Autodesk Fusion 360 part; units mm, degrees
sketch "Skizze1" plane through (0, 0, 0) normal (0, 0, 1) x (1, 0, 0)
  line L0 (-31.5508, 0) -> (33.8224, 0) construction
  line L1 (0, 25.6192) -> (0, -38.4919) construction
  circle A0 centre (0, 0) radius 1.75
  circle A1 centre (0, 0) radius 3.5
  circle A2 centre (0, 0) radius 5
  dimension "d1" = 3.5
  dimension "d2" = 7
  dimension "d3" = 10
extrude "Extrusion1" add sketch "Skizze1" along normal blind 7 contours A1 | A2
extrude "Extrusion2" add sketch "Skizze1" along normal blind 9.5 contours A1
ref_plane "Arbeitsebene1" through (0, 0, 3.5) normal (0, 0, 1) x (1, 0, 0)
sketch "Skizze2" plane through (0, 0, 3.5) normal (0, 0, 1) x (1, 0, 0)
  line L0 (-11, 0) -> (19, 0) construction
  line L1 (0, 16) -> (0, -23) construction
  line L2 (1.6743, -2.9) -> (3.3486, 0)
  line L3 (3.3486, 0) -> (1.6743, 2.9)
  line L4 (1.6743, 2.9) -> (-1.6743, 2.9)
  line L5 (-1.6743, 2.9) -> (-3.3486, 0)
  line L6 (-3.3486, 0) -> (-1.6743, -2.9)
  line L7 (-1.6743, -2.9) -> (1.6743, -2.9)
  dimension "d9" = 5.8
extrude "Extrusion3" cut sketch "Skizze2" along normal mid plane 2.8
Can you work these out from the model? Positions are in its coordinate system, mm. A direction names the side the tool comes from. Round coordinates to 2 decimals unless told otherwise and drop trailing zeros. Write each loop counter-clockwise with the first axis right and the second up, starting at its lowest first coordinate (ties: lowest second). Pieces come first, ordered by that corner, then holes. Notation, with made-up numbers: (85.5, 75) -> (129.5, 75) arc R24 ccw to (129.5, 96) -> close; hole circle Ø9 at (4, -9.75). An arc over 180 degrees is marked (long way). One line per question, with ' | ' between items. Start each with the question number.
1) I need wall thicknesses on line 1 (Y direction, x = 0, z = 0.65); line 2 (X direction, y = 0, z = 7.1). Which ranges of each line are inside material? Lowest first, please. Write a range as [from, to].
2) Suppose I cut it at D-D on x = -4. Write out the boundary of the cut face in (y, z), then the cut area to 3 significant figures.
3) If we mould it in two halves opening along Y, with no side actions, what happens to faces 4 (the flat face through (2, 0, 0)), 5 (the cylindrical face through (-1.08, 4.88, 3.45)), 6 (the flat face through (0, -2.9, 3))? For each: released by +Y, released by -Y, zero draft, split by the parting line, or undercut.
4) On a 3-axis mill with a long thin cutter (end or side, diameter ignored), from which of +Z, -Z, +X, -X, +Y, -Y can I reach the whole of each face in a straight line? I mean faces 1 (the flat face through (2.5, -1.47, 3.48)), 2 (the cylindrical face through (1.617, 0.67, 1.035)), 3 (the flat face through (2.2, -3.3, 7)). Say none if no direction works.
5) Suppose I cut it at C-C on y = -0.75. Write out the boundary of the cut face in (x, z), then the cut area to 3 significant figures.
6) Suppose I cut it at A-A on x = 0. Write out the boundary of the cut face in (y, z).
7) I'm going to push flat-ended pins straight in: P1, Ø1, axis at x = 3, y = 3, coming from the +Z side; P2, Ø3, axis at x = -2, z = 6, coming from the -Y side; P3, Ø2, axis at x = 3.5, z = 3.5, coming from the +Y side. Where does each tip first touch, or does it pass through?
8) Suppose I cut it at B-B on z = 4.75. Write out the boundary of the cut face in (x, y).
Return value:
1) line 1: y = [-5, -1.75], [1.75, 5] | line 2: x = [-3.5, -1.75], [1.75, 3.5]
2) outline: (-3, 0) -> (3, 0) -> (3, 7) -> (-3, 7) -> close | area: 42.0 mm2
3) face 4: zero draft | face 5: split by the parting line | face 6: undercut
4) face 1: none | face 2: +Z, -Z | face 3: +Z
5) outline: (-4.94, 0) -> (-1.58, 0) -> (-1.58, 2.1) -> (-2.92, 2.1) -> (-2.92, 4.9) -> (-1.58, 4.9) -> (-1.58, 9.5) -> (-3.42, 9.5) -> (-3.42, 7) -> (-4.94, 7) -> close; (1.58, 0) -> (4.94, 0) -> (4.94, 7) -> (3.42, 7) -> (3.42, 9.5) -> (1.58, 9.5) -> (1.58, 4.9) -> (2.92, 4.9) -> (2.92, 2.1) -> (1.58, 2.1) -> close | area: 48.8 mm2
6) outline: (-5, 0) -> (-1.75, 0) -> (-1.75, 2.1) -> (-2.9, 2.1) -> (-2.9, 4.9) -> (-1.75, 4.9) -> (-1.75, 9.5) -> (-3.5, 9.5) -> (-3.5, 7) -> (-5, 7) -> close; (1.75, 0) -> (5, 0) -> (5, 7) -> (3.5, 7) -> (3.5, 9.5) -> (1.75, 9.5) -> (1.75, 4.9) -> (2.9, 4.9) -> (2.9, 2.1) -> (1.75, 2.1) -> close
7) P1: stops at z = 7 | P2: stops at y = -4.97 | P3: stops at y = 4.33
8) outline: circle Ø10 at (0, 0); hole (-3.35, 0) -> (-1.67, -2.9) -> (1.67, -2.9) -> (3.35, 0) -> (1.67, 2.9) -> (-1.67, 2.9) -> close
